from build123d import *

# Parameters (mm, degrees)
F0_R     = 58.8324156358
F1_DEPTH = 63.5
F2_R     = 40.5716909801
F3_DEPTH = 63.501
F5_DEPTH = 25.4
F7_DEPTH = 12.7


with BuildPart() as f1:
    # F0 (on Top) → F1 (new body)
    with BuildSketch(Plane.XY):
        with Locations((78.2794505358, 0)):
            Circle(F0_R)
    extrude(amount=F1_DEPTH)

    # F2 (on Top) → F3 (cut, through all)
    with BuildSketch(Plane.XY):
        with Locations((77.139608562, 0)):
            Circle(F2_R)
    extrude(amount=F3_DEPTH, mode=Mode.SUBTRACT)

    # F4 (on Top) → F5 (join)
    with BuildSketch(Plane.XY):
        with BuildLine():
            add(Edge.make_bspline(
                [(-50.2571389079, -56.1054311693), (-16.7832059207, -55.6967128398), (32.1861465243, -55.0987946945), (67.1425862644, -57.641467666), (45.7816152555, -51.1111653509), (33.0959452068, -41.131486421), (22.5874521406, -22.5952197622), (18.4327377492, -5.9917502981), (19.0387832668, 11.3825225281), (25.1956842548, 27.0460198571), (30.7814993553, 37.5243375445), (45.4991432323, 49.5310228176), (55.0799139421, 54.1549944447), (59.7038790584, 56.3866607845)],
                knots=[0, 0, 0, 0, 0.1891612959, 0.2767259579, 0.3472655422, 0.4317314301, 0.5218364542, 0.6040854661, 0.6864673203, 0.766880288, 0.8353517069, 0.920535833, 1, 1, 1, 1], degree=3))
            Line((59.7038790584, 56.3866607845), (-50.2571389079, 56.3866607845))
            Line((-50.2571389079, 56.3866607845), (-50.2571389079, -56.1054311693))
        make_face()
    extrude(amount=F5_DEPTH)

    # F6 (on Front) → F7 (join)
    with BuildSketch(Plane.XZ):
        Polygon((19.521009177, 26.206118986), (19.521009177, 63.1586238742), (-24.5204272107, 26.206118986), align=None)
    extrude(amount=-F7_DEPTH)


solid = f1.part
The listing builds one solid part. Answer for the finished solid, in the listing's coordinates (mm). A direction names the side the tool comes from. Coordinates: 2 decimals unless noted, no trailing zeros. Order: outer loops, then holes, each group sorted by start corner. A loop starts at its lowest first (then second) coordinate and runs counter-clockwise, first axis right, second up. Notation, with made-up numbers: (66, -23) -> (75, -23) arc R19 ccw to (75, 1) -> close; hole circle Ø8 at (35, 6.25). An arc over 180 degrees is marked (long way). Answer in a Markdown table with one row per item. Add a question column.
Item 1: Find section C-C (y = -31.5). State how many separate pieces and enclosed holes the cut face has, then the cut area to 3 significant figures.
Item 2: Find the intervals of material crossed by L1, parallel to X at y = -18, z = 16; L2, parallel to Y at x = 108, z = 54.5; L3, parallel to Z at x = 23, y = -53, in increasing order. Write a range as from..to.
Item 3: Find section B-B (z = 33). Write down the section's boundary in (x, y), then the cut area to 3 significant figures.
Item 4: Each of these flat-tipped pins is pushed along its axis until it touches: P1, Ø3, axis at y = 5.5, z = 45.5, coming from the +X side; P2, Ø1, axis at y = -20, z = 18.5, coming from the +X side; P3, Ø1.5, axis at x = 101.5, z = 45.5, coming from the +Y side. Where does it stop, or does it pass through?
Item 5: Find section A-A (x = 83). Write down the section's boundary in (y, z), then the cut area to 3 significant figures.
Item 6: Which of the six approach directions +Z, -Z, +X, -X, +Y, -Y give full straight-line access (tool end or side, diameter ignored) to faces 4 (the face through (7, 0, 37)), 5 (the face through (-3, 6, 26.206)), 6 (the face through (5, 56.387, 13))?
Item 7: Determine the mould class of faces 1 (the face through (132.626, -22.533, 31.306)), 2 (the face through (-8, 0, 25.4)), 3 (the face through (7, 12.7, 37)) for opening direction Y: +Y half, -Y half, draft (parallel to the pull), parting line (faces both ways), or undercut.
Result set:
| question | item | result |
|---|---|---|
| 1 | separate pieces | 3 |
| 1 | enclosed holes | 0 |
| 1 | area | 5,050 mm² |
| 2 | L1 | x = -50.26..21.82, 22.27..40.78, 113.5..134.29 |
| 2 | L2 | y = -50.77..-26.34, 26.34..50.77 |
| 2 | L3 | z = 0..25.4 |
| 3 | outline | (-16.42, 0) -> (19.45, 0) arc R58.83 ccw (long way) to (19.52, 2.95) -> (19.52, 12.7) -> (-16.42, 12.7) -> close; hole circle Ø81.14 at (77.14, 0) |
| 3 | area | 6,160 mm² |
| 4 | P1 | stops at x = 136.98 |
| 4 | P2 | stops at x = 133.79 |
| 4 | P3 | stops at y = 54.37 |
| 5 | outline | (-58.64, 0) -> (-40.15, 0) -> (-40.15, 63.5) -> (-58.64, 63.5) -> close; (40.15, 0) -> (58.64, 0) -> (58.64, 63.5) -> (40.15, 63.5) -> close |
| 5 | area | 2,350 mm² |
| 6 | face 4 | +Z, -X, -Y |
| 6 | face 5 | -X, +Y, -Y |
| 6 | face 6 | +Z, -Z, -X, +Y |
| 7 | face 1 | undercut |
| 7 | face 2 | draft |
| 7 | face 3 | +Y half |
